from build123d import *

# Parameters (mm, degrees)
F0_W     = 5
F0_H     = 5
F1_DEPTH = 25


with BuildPart() as f1:
    # F0 (on Front) → F1 (new body)
    with BuildSketch(Plane.XZ):
        with BuildLine():
            ThreePointArc((35, 150.8578643763), (42.2474487139, 156.3397459622), (45, 165))
            ThreePointArc((45, 165), (21.3397459622, 177.2474487139), (25, 150.8578643763))
            ThreePointArc((25, 150.8578643763), (27.4634703191, 150.2160216052), (30, 150))
            ThreePointArc((30, 150), (32.5365296809, 150.2160216052), (35, 150.8578643763))
        make_face()
        with BuildLine():
            ThreePointArc((30, 150), (27.4634703191, 150.2160216052), (25, 150.8578643763))
            Line((25, 150.8578643763), (25, 145))
            Line((25, 145), (30, 145))
            Line((30, 145), (30, 150))
        make_face()
        with BuildLine():
            Line((35, 145), (35, 150.8578643763))
            ThreePointArc((35, 150.8578643763), (32.5365296809, 150.2160216052), (30, 150))
            Line((30, 150), (30, 145))
            Line((30, 145), (35, 145))
        make_face()
        with BuildLine():
            Line((25, 140), (25, 145))
            Line((25, 145), (5, 145))
            ThreePointArc((5, 145), (8.5355339059, 143.5355339059), (10, 140))
            Line((10, 140), (25, 140))
        make_face()
        with BuildLine():
            Line((30, 145), (25, 145))
            Line((25, 145), (25, 140))
            ThreePointArc((25, 140), (26.4644660941, 143.5355339059), (30, 145))
        make_face()
        with BuildLine():
            Line((35, 140), (35, 145))
            Line((35, 145), (30, 145))
            ThreePointArc((30, 145), (33.5355339059, 143.5355339059), (35, 140))
        make_face()
        with BuildLine():
            Line((55, 145), (35, 145))
            Line((35, 145), (35, 140))
            Line((35, 140), (50, 140))
            ThreePointArc((50, 140), (51.4644660941, 143.5355339059), (55, 145))
        make_face()
        with BuildLine():
            ThreePointArc((10, 140), (8.5355339059, 143.5355339059), (5, 145))
            ThreePointArc((5, 145), (1.4644660941, 143.5355339059), (0, 140))
            ThreePointArc((0, 140), (1.4644660941, 136.4644660941), (5, 135))
            Line((5, 135), (5, 140))
            Line((5, 140), (10, 140))
        make_face()
        with BuildLine():
            ThreePointArc((30, 135), (26.4644660941, 136.4644660941), (25, 140))
            Line((25, 140), (10, 140))
            Line((10, 140), (10, 135))
            Line((10, 135), (15, 135))
            Line((15, 135), (30, 135))
        make_face()
        with BuildLine():
            ThreePointArc((60, 140), (58.5355339059, 143.5355339059), (55, 145))
            ThreePointArc((55, 145), (51.4644660941, 143.5355339059), (50, 140))
            Line((50, 140), (55, 140))
            Line((55, 140), (55, 135))
            ThreePointArc((55, 135), (58.5355339059, 136.4644660941), (60, 140))
        make_face()
        with BuildLine():
            Line((50, 140), (35, 140))
            ThreePointArc((35, 140), (33.5355339059, 136.4644660941), (30, 135))
            Line((30, 135), (45, 135))
            Line((45, 135), (50, 135))
            Line((50, 135), (50, 140))
        make_face()
        with BuildLine():
            ThreePointArc((5, 135), (1.4644660941, 136.4644660941), (0, 140))
            Line((0, 140), (0, 80))
            ThreePointArc((0, 80), (5, 75), (10, 80))
            Line((10, 80), (10, 135))
            Line((10, 135), (5, 135))
        make_face()
        with Locations((7.5, 137.5)):
            Rectangle(F0_W, F0_H)
        with BuildLine():
            Line((45, 135), (30, 135))
            Line((30, 135), (30, 75))
            Line((30, 75), (35, 75))
            ThreePointArc((35, 75), (40, 80), (45, 75))
            Line((45, 75), (45, 135))
        make_face()
        with BuildLine():
            Line((30, 75), (30, 135))
            Line((30, 135), (15, 135))
            Line((15, 135), (15, 75))
            ThreePointArc((15, 75), (20, 80), (25, 75))
            Line((25, 75), (30, 75))
        make_face()
        with BuildLine():
            Line((60, 80), (60, 140))
            ThreePointArc((60, 140), (58.5355339059, 136.4644660941), (55, 135))
            Line((55, 135), (50, 135))
            Line((50, 135), (50, 80))
            ThreePointArc((50, 80), (55, 75), (60, 80))
        make_face()
        with Locations((52.5, 137.5)):
            Rectangle(F0_W, F0_H)
        Polygon((35, 75), (30, 75), (25, 75), (25, 70), (30, 70), (35, 70), align=None)
        with BuildLine():
            Line((25, 70), (25, 75))
            ThreePointArc((25, 75), (20, 80), (15, 75))
            Line((15, 75), (15, 5))
            ThreePointArc((15, 5), (20, 0), (25, 5))
            Line((25, 5), (25, 70))
        make_face()
        with BuildLine():
            ThreePointArc((45, 75), (40, 80), (35, 75))
            Line((35, 75), (35, 70))
            Line((35, 70), (35, 5))
            ThreePointArc((35, 5), (40, 0), (45, 5))
            Line((45, 5), (45, 75))
        make_face()
        with BuildLine():
            ThreePointArc((35, 140), (33.5355339059, 143.5355339059), (30, 145))
            Line((30, 145), (30, 140))
            Line((30, 140), (35, 140))
        make_face()
        with BuildLine():
            Line((30, 140), (30, 145))
            ThreePointArc((30, 145), (26.4644660941, 143.5355339059), (25, 140))
            Line((25, 140), (30, 140))
        make_face()
        with BuildLine():
            Line((30, 140), (25, 140))
            ThreePointArc((25, 140), (26.4644660941, 136.4644660941), (30, 135))
            Line((30, 135), (30, 140))
        make_face()
        with BuildLine():
            ThreePointArc((30, 135), (33.5355339059, 136.4644660941), (35, 140))
            Line((35, 140), (30, 140))
            Line((30, 140), (30, 135))
        make_face()
    extrude(amount=F1_DEPTH)


solid = f1.part
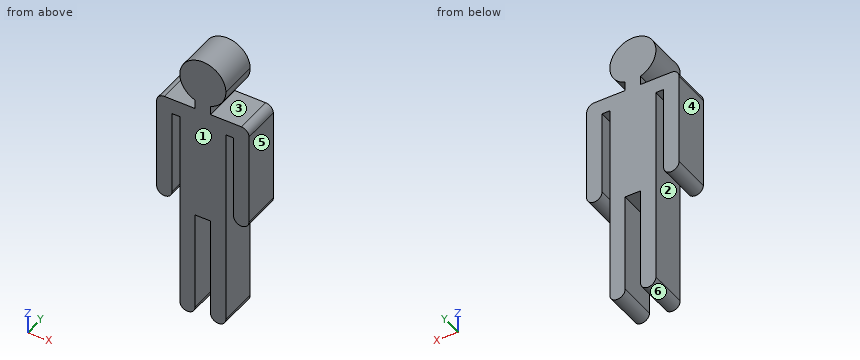
Check sheet for the modelled part. Datum: model origin and axes. Units: mm. Face numbers are marked on the shaded views. A direction names the side the tool comes from. Round coordinates to 2 decimals unless told otherwise and drop trailing zeros. Order: outer loops, then holes, each group sorted by start corner. A loop starts at its lowest first (then second) coordinate and runs counter-clockwise, first axis right, second up.
(1) Cross-section at C-C, the plane y = -4. Enter the section's corners in (x, z), and give its area (3 significant figures).
(2) Cross-section at D-D, the plane x = 30. Enter the section's corners in (y, z).
(3) Cross-section at A-A, the plane z = 19. Enter the section's corners in (x, y), and give its area (3 significant figures).
(4) Go/stop test with flat-tipped pins: P1, Ø6.5, axis at y = -14, z = 149.5, coming from the +X side; P2, Ø2, axis at x = 52, y = -16.5, coming from the +Z side; P3, Ø6, axis at x = 29.5, y = -17.5, coming from the -Z side. Record where each tip stops, or that it passes through.
(5) Cross-section at B-B, the plane x = 20. Enter the section's corners in (y, z).
(6) Scan lines: probe 1 along X at (y, z) = (-11.5, 84.5); probe 2 along X at (y, z) = (-17.5, 59); probe 3 along Z at (x, y) = (47, -13.25). Record each from-to range of solid material in increasing order.
(7) Draft check along X on the marked faces 3, 4, 5 and 6. Enter one of: pulls with the +X half, pulls with the -X half, needs draft (parallel to the pull), parting line crosses it, or undercut.
(8) Access from +Z, -Z, +X, -X, +Y, -Y to the whole of each face (thin tool, end or side, straight path). Record for the marked faces 1 and 2.
Check sheet entries:
1. outline: (0, 80) arc R5 ccw to (10, 80) - (10, 135) - (15, 135) - (15, 5) arc R5 ccw to (25, 5) - (25, 70) - (35, 70) - (35, 5) arc R5 ccw to (45, 5) - (45, 135) - (50, 135) - (50, 80) arc R5 ccw to (60, 80) - (60, 140) arc R5 ccw to (55, 145) - (35, 145) - (35, 150.86) arc R15 ccw (long way) to (25, 150.86) - (25, 145) - (5, 145) arc R5 ccw to (0, 140) - close
1. area: 5,860 mm2
2. outline: (-25, 70) - (0, 70) - (0, 180) - (-25, 180) - close
3. outline: (15, -25) - (25, -25) - (25, 0) - (15, 0) - close; (35, -25) - (45, -25) - (45, 0) - (35, 0) - close
3. area: 500 mm2
4. P1: stops at x = 38.66
4. P2: stops at z = 145
4. P3: stops at z = 70
5. outline: (-25, 0) - (0, 0) - (0, 145) - (-25, 145) - close; (-25, 153.82) - (0, 153.82) - (0, 176.18) - (-25, 176.18) - close
6. probe 1: x = 0 to 10, 15 to 45, 50 to 60
6. probe 2: x = 15 to 25, 35 to 45
6. probe 3: z = 135 to 145
7. face 3: needs draft
7. face 4: pulls with the -X half
7. face 5: pulls with the +X half
7. face 6: undercut
8. face 1: +Z, -Z, +X, -X, -Y
8. face 2: -Z, +Y, -Y
